For this review, take the finished solid that the model builds, in its own axes (mm). A direction names the side the tool comes from. Round coordinates to 2 decimals unless told otherwise and drop trailing zeros. Write each loop counter-clockwise with the first axis right and the second up, starting at its lowest first coordinate (ties: lowest second). Pieces come first, ordered by that corner, then holes. Notation, with made-up numbers: M -11.75,-39.5 L 11.25,-39.5 A17 ccw 11.25,-24.5 Z; hole C -34,-3 d6. An arc over 180 degrees is marked long. Use one line per item in the form item = value. Start each with the question number.
Item 1: Add section D-D (x = 3.25). State the section outline as (y, z) points, and give its area (3 significant figures).
Item 2: Add section A-A (x = 0). State the section outline as (y, z) points, and give its area (3 significant figures).
Item 3: Add section B-B (z = 3.5). State the section outline as (x, y) points, and give its area (3 significant figures).
Item 4: For line 1 (Y direction, x = 0, z = 0.4); line 2 (X direction, y = 0, z = 0.25); line 3 (X direction, y = 0, z = 2.75), list the stretches that pass through material, from the lowest coordinate up. Write a range as [from, to].
Item 5: For P1, Ø1.5, axis at x = 4.5, y = -5, coming from the +Z side; P2, Ø3, axis at y = -5, z = 2.5, coming from the -X side, all flat-tipped, find the tip position at first contact; note any pin that passes through.
Item 6: Add section C-C (y = 1.5). State the section outline as (x, z) points.
Item 7: Draft analysis for pull direction Y (two halves, no side actions). For faces 5 (the cylindrical face through (6.583, -2.073, 0.246)), 6 (the flat face through (0, 4, 2.9)), 7 (the cylindrical face through (-0.18, -4.246, 4.773)), 8 (the flat face through (-0.373, 7.757, 1.47)), state which applies: released by +Y, released by -Y, zero draft, split by the parting line, or undercut.
Item 8: For faces 1 (the flat face through (0.37, 7.74, 1.47)), 2 (the cylindrical face through (-1.063, 4.785, 0.246)), 3 (the flat face through (-2, -7, 0)), 4 (the flat face through (0.367, 3.739, 4.827)), list the 3-axis set-ups (+Z, -Z, +X, -X, +Y, -Y) from which the entire face can be reached by the end or side of a thin tool; tool diameter is ignored.
from build123d import *

# Parameters (mm, degrees)
F0_R      = 8.25
F1_DEPTH  = 2.9
F2_R      = 4.25
F3_DEPTH  = 3.8
F5_DEPTH  = 2.9
F7_DEPTH  = 3.8
F8_R      = 2.25
F9_DEPTH  = 6.7
F8_R_2    = 6.9020481578
F8_R_3    = 4.9020481578
F8_R_4    = 3.9020481578
F8_R_5    = 2.9020481578
F10_DEPTH = 0.5


with BuildPart() as f1:
    # F0 (on Top) → F1 (new body)
    with BuildSketch(Plane.XY):
        Circle(F0_R)
    extrude(amount=F1_DEPTH)

    # F2 (on face) → F3 (join)
    with BuildSketch(Plane.XY.offset(2.9)):
        Circle(F2_R)
    extrude(amount=F3_DEPTH)

    # F4 (on face) → F5 (cut)
    with BuildSketch(Plane.XY.offset(2.9)):
        with BuildLine():
            ThreePointArc((0.4919195185, 8.2353211952), (0, 8.25), (-0.4919195185, 8.2353211952))
            Line((-0.4919195185, 8.2353211952), (-0.25, 7.265035003))
            Line((-0.25, 7.265035003), (0.25, 7.265035003))
            Line((0.25, 7.265035003), (0.4919195185, 8.2353211952))
        make_face()
    extrude(amount=-F5_DEPTH, mode=Mode.SUBTRACT)

    # F6 (on face) → F7 (cut)
    with BuildSketch(Plane.XY.offset(6.7)):
        with BuildLine():
            ThreePointArc((0.4875978882, 4.221936558), (0, 4.25), (-0.4875978882, 4.221936558))
            Line((-0.4875978882, 4.221936558), (-0.25, 3.2689834782))
            Line((-0.25, 3.2689834782), (0.25, 3.2689834782))
            Line((0.25, 3.2689834782), (0.4875978882, 4.221936558))
        make_face()
    extrude(amount=-F7_DEPTH, mode=Mode.SUBTRACT)

    # F8 (on face) → F9 (cut)
    with BuildSketch(Plane(origin=(0, 0, 0), x_dir=(1, 0, 0), z_dir=(0, 0, -1))):
        Circle(F8_R)
    extrude(amount=-F9_DEPTH, mode=Mode.SUBTRACT)

    # F8 (on face) → F10 (cut)
    with BuildSketch(Plane(origin=(0, 0, 0), x_dir=(1, 0, 0), z_dir=(0, 0, -1))):
        Circle(F8_R_2)
        Circle(F8_R_3, mode=Mode.SUBTRACT)
        Circle(F8_R_4)
        Circle(F8_R_5, mode=Mode.SUBTRACT)
    extrude(amount=-F10_DEPTH, mode=Mode.SUBTRACT)


solid = f1.part
Calculated:
q1.outline = M -7.58,0 L -6.09,0 L -6.09,0.5 L -3.67,0.5 L -3.67,0 L -2.16,0 L -2.16,0.5 L 2.16,0.5 L 2.16,0 L 3.67,0 L 3.67,0.5 L 6.09,0.5 L 6.09,0 L 7.58,0 L 7.58,2.9 L 2.74,2.9 L 2.74,6.7 L -2.74,6.7 L -2.74,2.9 L -7.58,2.9 Z
q1.area = 60.2 mm^2
q2.outline = M -8.25,0 L -6.9,0 L -6.9,0.5 L -4.9,0.5 L -4.9,0 L -3.9,0 L -3.9,0.5 L -2.9,0.5 L -2.9,0 L -2.25,0 L -2.25,6.7 L -4.25,6.7 L -4.25,2.9 L -8.25,2.9 Z; M 2.25,0 L 2.9,0 L 2.9,0.5 L 3.9,0.5 L 3.9,0 L 4.9,0 L 4.9,0.5 L 6.9,0.5 L 6.9,0 L 7.27,0 L 7.27,2.9 L 3.27,2.9 L 3.27,6.7 L 2.25,6.7 Z
q2.area = 40.4 mm^2
q3.outline = M -0.49,4.22 A4.25 ccw long 0.49,4.22 L 0.25,3.27 L -0.25,3.27 Z; hole C 0,0 d4.5
q3.area = 40.1 mm^2
q4.line_1 = [-8.25, -6.9], [-4.9, -3.9], [-2.9, -2.25], [2.25, 2.9], [3.9, 4.9], [6.9, 7.27]
q4.line_2 = [-8.25, -6.9], [-4.9, -3.9], [-2.9, -2.25], [2.25, 2.9], [3.9, 4.9], [6.9, 8.25]
q4.line_3 = [-8.25, -2.25], [2.25, 8.25]
q5.P1 = 2.9
q5.P2 = -7.47
q6.outline = M -8.11,0 L -6.74,0 L -6.74,0.5 L -4.67,0.5 L -4.67,0 L -3.6,0 L -3.6,0.5 L -2.48,0.5 L -2.48,0 L -1.68,0 L -1.68,6.7 L -3.98,6.7 L -3.98,2.9 L -8.11,2.9 Z; M 1.68,0 L 2.48,0 L 2.48,0.5 L 3.6,0.5 L 3.6,0 L 4.67,0 L 4.67,0.5 L 6.74,0.5 L 6.74,0 L 8.11,0 L 8.11,2.9 L 3.98,2.9 L 3.98,6.7 L 1.68,6.7 Z
q7.face_5 = undercut
q7.face_6 = zero draft
q7.face_7 = split by the parting line
q7.face_8 = released by +Y
q8.face_1 = +Z, -Z, +Y
q8.face_2 = -Z
q8.face_3 = -Z, +X, -X, +Y, -Y
q8.face_4 = +Z, +Y
